Can you work these out from the model? Positions are in its coordinate system, mm. Face numbers are marked on the shaded views. A direction names the side the tool comes from. Give positions to 0.01 mm unless a question says otherwise; leave off trailing zeros. Loops run counter-clockwise (first coordinate to the right, second up) from the corner with the lowest first, then second, coordinate; pieces in that order, holes last. Notation, with made-up numbers: M 50.5,11.5 L 105.5,11.5 A33 ccw 105.5,50.5 Z; hole C 28.5,-40 d9. An arc over 180 degrees is marked long. Answer as a JSON object with one key per item and string values.
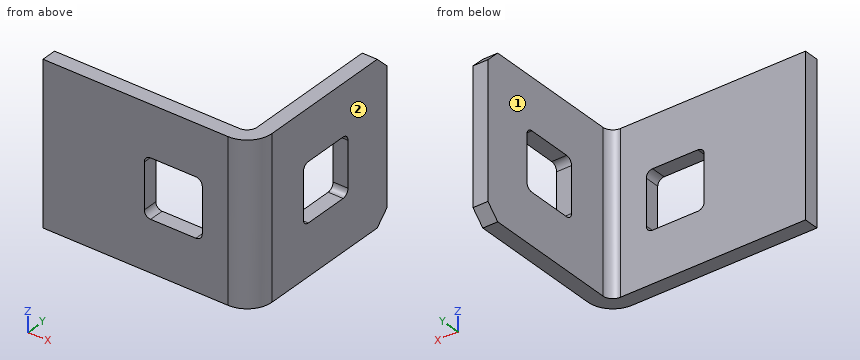
Autodesk Inventor part; units mm, degrees
ref_plane "Flange Pattern Plane" through (31.75, 7.5406, -4.5466) normal (0, 1, 0) x (1, 0, 0)
ref_plane "YZ Plane" through (0, 0, 0) normal (1, 0, 0) x (0, 1, 0)
ref_plane "XZ Plane" through (0, 0, 0) normal (0, 1, 0) x (-1, 0, 0)
sketch "Sketch1" plane through (0, 0, 0) normal (0, 1, 0) x (-1, 0, 0)
  line L0 (-31.75, 0) -> (31.75, 0)
  line L1 (31.75, 0) -> (31.75, -12.7)
  line L2 (31.75, -12.7) -> (-31.75, -12.7)
  line L3 (-31.75, -12.7) -> (-31.75, 0)
  line L4 (31.75, 0) -> (-31.75, -12.7) construction
  point P0 (0, 0)
  point P1 (0, 0)
  dimension "d0" = 63.5
  dimension "d1" = 12.7
extrude "Plate1" add sketch "Sketch1" along normal blind 1.1906
sketch "Sketch2" plane through (30.5594, 0, -12.7) normal (1, 0, 0) x (0, 1, 0)
  line L0 (0, 12.7) -> (0, 0)
  line L1 (0, 0) -> (13.8906, 0)
  line L2 (13.8906, 0) -> (13.8906, 12.7)
  line L3 (13.8906, 12.7) -> (0, 12.7)
edge flange "Flanges" height 12.7 angle 90 thickness 1.1906 bend radius 0.7937 thickness toward (1, 0, 0) relief tear relief width 1.1906 relief depth 0.5953 corner gap 1.1906 corner form 0 edges at (31.75, 1.1906, -6.35) (-31.75, 1.1906, -6.35) wall of the first edge with corners at (30.5594, 0, 0) (30.5594, 0, -12.7) (30.5594, 13.8906, -12.7) (30.5594, 13.8906, 0)
bend "Bend1"
corner "Corner1"
sketch "Sketch3" plane through (31.75, 1.9844, -12.7) normal (1, 0, 0) x (0, 0, -1)
  line L0 (-8.1534, 7.8677) -> (-4.5466, 7.8677)
  line L1 (-4.0386, 7.3597) -> (-4.0386, 3.7529)
  line L2 (-4.5466, 3.2449) -> (-8.1534, 3.2449)
  line L3 (-8.6614, 3.7529) -> (-8.6614, 7.3597)
  arc A0 (-8.1534, 7.8677) -> (-8.6614, 7.3597) centre (-8.1534, 7.3597) ccw
  arc A1 (-4.0386, 7.3597) -> (-4.5466, 7.8677) centre (-4.5466, 7.3597) ccw
  arc A2 (-4.5466, 3.2449) -> (-4.0386, 3.7529) centre (-4.5466, 3.7529) ccw
  arc A3 (-8.6614, 3.7529) -> (-8.1534, 3.2449) centre (-8.1534, 3.7529) ccw
  line L4 (-12.7, 0) -> (-12.7, 11.9063) construction
  line L5 (-12.7, 11.9063) -> (0, 11.9063) construction
  line L6 (-8.1534, 7.3597) -> (-4.5466, 3.7529) construction
  point P0 (-12.7, -1.9844)
  point P1 (-4.0386, 3.2449)
  point P2 (-8.6614, 3.2449)
  point P3 (-6.35, 5.5563)
  dimension "d16" = 4.6228
  dimension "d17" = 0.508
  dimension "d20" = 6.35
  dimension "d21" = 6.35
extrude "Flange Stamp" cut sketch "Sketch3" against normal blind 1.1906
sketch "Sketch7" plane through (31.75, 1.9844, 0) normal (1, 0, 0) x (0, 0, -1)
  arc A0 (4.5466, 7.8677) -> (4.0386, 7.3597) centre (4.5466, 7.3597) ccw construction
  arc A1 (8.1534, 3.2449) -> (8.6614, 3.7529) centre (8.1534, 3.7529) ccw construction
  circle A2 centre (6.35, 5.5563) radius 2.1844
  line L0 (4.5466, 7.3597) -> (8.1534, 3.7529) construction
  point P0 (0, -1.9844)
  dimension "d46" = 4.3688
surface extrude "Flange Circle" sketch "Sketch7" against normal up to surface (1.1906 mm away) shown yes curves A2
ref_plane "Flange Pattern Plane" through (31.75, 7.5406, -4.5466) normal (0, 1, 0) x (1, 0, 0)
feature "Flange Pattern" [suppressed]
sketch "Sketch8" plane through (0, 0, 0) normal (0, -1, 0) x (1, 0, 0)
  line L0 (29.7656, 0) -> (-29.7656, 0) construction
  line L1 (27.2034, -4.0386) -> (23.5966, -4.0386)
  line L2 (23.0886, -4.5466) -> (23.0886, -8.1534)
  line L3 (23.5966, -8.6614) -> (27.2034, -8.6614)
  line L4 (27.7114, -8.1534) -> (27.7114, -4.5466)
  arc A0 (27.7114, -4.5466) -> (27.2034, -4.0386) centre (27.2034, -4.5466) ccw
  arc A1 (27.2034, -8.6614) -> (27.7114, -8.1534) centre (27.2034, -8.1534) ccw
  arc A2 (23.0886, -8.1534) -> (23.5966, -8.6614) centre (23.5966, -8.1534) ccw
  arc A3 (23.5966, -4.0386) -> (23.0886, -4.5466) centre (23.5966, -4.5466) ccw
  line L5 (27.2034, -4.5466) -> (23.5966, -8.1534) construction
  line L6 (31.75, 0) -> (31.75, -12.7) construction
  point P0 (0, 0)
  point P1 (23.0886, -8.6614)
  point P2 (27.7114, -8.6614)
  point P3 (25.4, -6.35)
  dimension "d49" = 4.6228
  dimension "d50" = 0.508
  dimension "d51" = 6.35
  dimension "d52" = 6.35
extrude "Body Stamp" cut sketch "Sketch8" against normal blind 1.1906
sketch "Sketch9" plane through (0, 0, 0) normal (0, -1, 0) x (1, 0, 0)
  arc A0 (27.7114, -4.5466) -> (27.2034, -4.0386) centre (27.2034, -4.5466) ccw construction
  arc A1 (23.0886, -8.1534) -> (23.5966, -8.6614) centre (23.5966, -8.1534) ccw construction
  line L0 (27.2034, -4.5466) -> (23.5966, -8.1534) construction
  circle A2 centre (25.4, -6.35) radius 2.1844
  point P0 (0, 0)
  dimension "d55" = 4.3688
surface extrude "Body Circle" sketch "Sketch9" against normal up to surface (1.1906 mm away) shown yes curves A2
feature "Body Pattern" [suppressed]
sketch "Arc Length" plane through (30.5594, 1.9844, 0) normal (0, 0, 1) x (1, 0, 0)
  line L0 (0, 0) -> (1.1906, 0) construction
  arc A0 (-0.7938, -0.7938) -> (0, 0) centre (-0.7938, 0) ccw construction
  line L1 (-0.7938, -1.9844) -> (-0.7938, -0.7938) construction
  arc A1 (-0.7938, -1.9844) -> (1.1906, 0) centre (-0.7938, 0) ccw construction
  point P0 (-30.5594, -1.9844)
  dimension "d85" = 3.117
  dimension "d92" = 1.2468
sketch "Sketch13" plane through (31.75, 13.8906, 0) normal (1, 0, 0) x (0, 0, -1)
  line L0 (0, 0) -> (12.7, 0) construction
  line L1 (62.4078, 0) -> (63.4238, -1.016)
  line L2 (63.4238, -1.016) -> (64.4398, 0)
  line L3 (62.4078, 0) -> (64.4398, 0)
  line L4 (12.7, -11.9063) -> (0, -11.9063) construction
  line L5 (63.4238, -10.8903) -> (61.3168, -12.9972)
  line L6 (61.3168, -12.9972) -> (63.4238, -15.1042)
  line L7 (63.4238, -15.1042) -> (65.5308, -12.9972)
  line L8 (65.5308, -12.9972) -> (63.4238, -10.8903)
  line L9 (63.4238, -10.8903) -> (63.4238, -15.1042) construction
  line L10 (63.4238, -1.016) -> (63.4238, -10.8903) construction
  line L11 (0, -11.9063) -> (12.7, -11.9063) construction
  point P0 (0, -13.8906)
  dimension "d86" = 4.2139
  dimension "d88" = 1.016
  dimension "d91" = 1.016
  dimension "d102" = 63.4238
feature "Notch" [suppressed]
mirror "Notch Mirror" [suppressed]
pattern_linear "Notch Pattern" [suppressed]
chamfer "End Chamfer" distance 1.016 angle 45 4 edges at (-31.1547, 13.8906, -12.7) (31.1547, 13.8906, -12.7) (-31.1547, 13.8906, 0) (31.1547, 13.8906, 0)
sketch "Sketch14" plane through (-31.75, 1.9844, 431.8) normal (1, 0, 0) x (0, 0, -1)
  line L0 (431.8, 11.9063) -> (444.5, 11.9063) construction
  line L1 (431.8, 0) -> (431.8, 11.9063) construction
  line L2 (431.8, -1.9844) -> (444.5, -1.9844) construction
  line L3 (431.8, 11.9063) -> (444.5, 11.9063)
  line L4 (444.5, 11.9063) -> (444.5, -1.9844)
  line L5 (444.5, -1.9844) -> (431.8, -1.9844)
  line L6 (431.8, -1.9844) -> (431.8, 11.9063)
  point P0 (382.0521, -1.9844)
extrude "Half Cut" cut sketch "Sketch14" along normal blind 46.7614
sketch "Flange Pattern Sketch" plane through (31.75, 7.5406, -4.5466) normal (0, 1, 0) x (1, 0, 0)
  line L0 (0, 3.6068) -> (0, 0) construction
  line L1 (-76.2822, -4.5466) -> (13.1932, -4.5466) construction
  line L2 (0, 0) -> (-1.1906, 0) construction
  point P0 (-31.75, -4.5466)
  point P1 (0, 1.8034)
  point P2 (0, 14.5034)
  point P3 (0, 27.2034)
  point P4 (0, 39.9034)
  point P5 (0, 52.6034)
  point P6 (0, 65.3034)
  point P7 (0, 78.0034)
  point P8 (0, 90.7034)
  point P9 (0, 103.4034)
  point P10 (0, 116.1034)
  point P11 (0, 128.8034)
  point P12 (0, 141.5034)
  point P13 (0, 154.2034)
  point P14 (0, 166.9034)
  point P15 (0, 179.6034)
  point P16 (0, 192.3034)
  point P17 (0, 205.0034)
  point P18 (0, 217.7034)
  point P19 (0, 230.4034)
  point P20 (0, 243.1034)
  point P21 (0, 255.8034)
  point P22 (0, 268.5034)
  point P23 (0, 281.2034)
  point P24 (0, 293.9034)
  point P25 (0, 306.6034)
  point P26 (0, 319.3034)
  point P27 (0, 332.0034)
  point P28 (0, 344.7034)
  point P29 (0, 357.4034)
  point P30 (0, 370.1034)
  point P31 (0, 382.8034)
  point P32 (0, 395.5034)
  point P33 (0, 408.2034)
  point P34 (0, 420.9034)
  point P35 (0, 433.6034)
  dimension "d131" = 12.7
  dimension "d134" = 12.7
sketch "Body Pattern Sketch" plane through (0, 0, 0) normal (0, -1, 0) x (1, 0, 0)
  line L0 (29.7656, 0) -> (-29.7656, 0) construction
  line L1 (31.75, 0) -> (31.75, -12.7) construction
  circle A0 centre (25.4, -6.35) radius 2.1844 construction
  point P0 (0, 0)
  point P1 (25.4, -19.05)
  point P2 (25.4, -31.75)
  point P3 (25.4, -44.45)
  point P4 (25.4, -57.15)
  point P5 (25.4, -69.85)
  point P6 (25.4, -82.55)
  point P7 (25.4, -95.25)
  point P8 (25.4, -107.95)
  point P9 (25.4, -120.65)
  point P10 (25.4, -133.35)
  point P11 (25.4, -146.05)
  point P12 (25.4, -158.75)
  point P13 (25.4, -171.45)
  point P14 (25.4, -184.15)
  point P15 (25.4, -196.85)
  point P16 (25.4, -209.55)
  point P17 (25.4, -222.25)
  point P18 (25.4, -234.95)
  point P19 (25.4, -247.65)
  point P20 (25.4, -260.35)
  point P21 (25.4, -273.05)
  point P22 (25.4, -285.75)
  point P23 (25.4, -298.45)
  point P24 (25.4, -311.15)
  point P25 (25.4, -323.85)
  point P26 (25.4, -336.55)
  point P27 (25.4, -349.25)
  point P28 (25.4, -361.95)
  point P29 (25.4, -374.65)
  point P30 (25.4, -387.35)
  point P31 (25.4, -400.05)
  point P32 (25.4, -412.75)
  point P33 (25.4, -425.45)
  point P34 (25.4, -438.15)
  dimension "d62" = 12.7
  dimension "d65" = 12.7
  dimension "d139" = 12.7
equation "\"d1\" = 1.27 * Length"
equation "\"d18\" = Thickness"
equation "\"d53\" = Thickness"
equation "\"d89\" = Thickness"
equation "\"d2\" = Thickness"
equation "\"d3\" = BendReliefWidth"
equation "\"d4\" = BendReliefDepth"
equation "\"d5\" = MinimumRemnant"
equation "\"d6\" = TransitionRadius"
equation "\"d10\" = CornerReliefSize"
equation "\"d11\" = GapSize"
equation "\"d12\" = JacobiRadiusSize"
equation "\"BendRadius\" = Thickness"
equation "\"BendReliefWidth\" = Thickness"
equation "\"BendReliefDepth\" = 0.5 * Thickness"
equation "\"CornerReliefSize\" = 4 * Thickness"
equation "\"MinimumRemnant\" = 2 * Thickness"
equation "\"TransitionRadius\" = BendRadius"
equation "\"JacobiRadiusSize\" = BendRadius"
equation "\"GapSize\" = Thickness"
properties part number "Alu C 1x3x1x35"
1) Suppose I cut it at C-C, the plane z = -7. Write out the boundary of the cut face in (x, y), and give its area (3 significant figures).
Answer list:
{"outline": "M 15.01,0 L 23.09,0 L 23.09,1.19 L 15.01,1.19 Z; M 27.71,0 L 29.77,0 A1.98 ccw 31.75,1.98 L 31.75,5.23 L 30.56,5.23 L 30.56,1.98 A0.79 cw 29.77,1.19 L 27.71,1.19 Z; M 30.56,9.85 L 31.75,9.85 L 31.75,13.89 L 30.56,13.89 Z", "area": "23.3 mm^2"}
2) Please list where these lines run through material, in increasing order: line 1 along X through (y, z) = (4.5, -6); line 2 along Y through (x, z) = (17, -10.5); line 3 along Y through (x, z) = (30.75, -6). Write a range as from..to.
Answer list:
{"line 1": "30.56..31.75", "line 2": "0..1.19", "line 3": "0.26..5.23, 9.85..13.89"}
3) Suppose I cut it at D-D, the plane z = -3.5. Write out the boundary of the cut face in (x, y), and give its area (3 significant figures).
Answer list:
{"outline": "M 15.01,0 L 29.77,0 A1.98 ccw 31.75,1.98 L 31.75,13.89 L 30.56,13.89 L 30.56,1.98 A0.79 cw 29.77,1.19 L 15.01,1.19 Z", "area": "34.3 mm^2"}
4) Will these pins go through, and if not, where does the flat tip stop? pin 1 Ø4 at (x, z) = (20, -7.5) entering from +Y; pin 2 Ø1 at (y, z) = (8, -10.5) entering from -X.
Answer list:
{"pin 1": "y = 1.19", "pin 2": "x = 30.56"}
5) For the marked faces 1 and 2, which set-ups out of +Z, -Z, +X, -X, +Y, -Y let a thin tool reach every point of the face, with its end or its side?
Answer list:
{"face 1": "+Z, -Z, -X, +Y", "face 2": "+Z, -Z, +X, +Y, -Y"}
6) Suppose I cut it at B-B, the plane x = 24.75. Write out the boundary of the cut face in (y, z), and give its area (3 significant figures).
Answer list:
{"outline": "M 0,-12.7 L 1.19,-12.7 L 1.19,-8.66 L 0,-8.66 Z; M 0,-4.04 L 1.19,-4.04 L 1.19,0 L 0,0 Z", "area": "9.62 mm^2"}
7) Suppose I cut it at A-A, the plane y = 8.25. Write out the boundary of the cut face in (x, z).
Answer list:
{"outline": "M 30.56,-12.7 L 31.75,-12.7 L 31.75,-8.66 L 30.56,-8.66 Z; M 30.56,-4.04 L 31.75,-4.04 L 31.75,0 L 30.56,0 Z"}
